```python
from build123d import *

# Parameters (mm, degrees)
SKETCH1_R           = 2.286
BOSS_EXTRUDE1_DEPTH = 12.7
FILLET1_R           = 0.79375


with BuildPart() as part:
    # Sketch1 → Boss-Extrude1 (new body)
    with BuildSketch(Plane(origin=(0, 0, 0), x_dir=(1, 0, 0), z_dir=(0, 1, 0))):
        with BuildLine():
            Line((5.992681083, 6.35), (-5.992681083, 6.35))
            ThreePointArc((-5.992681083, 6.35), (0, -8.73125), (5.992681083, 6.35))
        make_face()
        with Locations(Location((0, 0, 0), (0, 0, 270))):
            Circle(SKETCH1_R, mode=Mode.SUBTRACT)
    extrude(amount=BOSS_EXTRUDE1_DEPTH)

    # Fillet1
    fillet1_edges = [part.edges().sort_by_distance(p)[0] for p in [
        (-5.992681083, 6.35, -6.35),
        (5.992681083, 6.35, -6.35),
        (0, 12.7, 8.73125),
        (0, 12.7, -6.35),
    ]]
    fillet(fillet1_edges, radius=FILLET1_R)


solid = part.part
```
The listing builds one solid part. Answer for the finished solid, in the listing's coordinates (mm). Round coordinates to 2 decimals unless told otherwise and drop trailing zeros. Loops run counter-clockwise (first coordinate to the right, second up) from the corner with the lowest first, then second, coordinate; pieces in that order, holes last. Notation, with made-up numbers: (78, 2.5) - (92, 2.5) arc R17 ccw to (92, 16.5) - close; hole circle Ø11 at (15.5, -15). An arc over 180 degrees is marked (long way). Return JSON: item names as keys, results as strings. Group by question number.
1. Consider probe 1 along X at (y, z) = (4.5, 0); probe 2 along X at (y, z) = (2.5, -0.75); probe 3 along Z at (x, y) = (-1, 2.5). Determine where each line is inside the solid, lowest interval first.
2. Each of these flat-tipped pins is pushed along its axis until it touches: P1, Ø6, axis at y = 4.5, z = -4.5, coming from the -X side; P2, Ø3, axis at x = 0.5, z = -0.5, coming from the -Y side; P3, Ø1, axis at x = -7, y = 9.5, coming from the +Z side; P4, Ø5, axis at y = 9, z = -4, coming from the +X side. Where does it stop, or does it pass through?
3. The part is cut by section B-B on y = 10.25. Determine the outline of the cut face in (x, z).
4. The part is cut by section A-A on x = 0. Determine the outline of the cut face in (y, z).
5. The mould has two halves that part along X. Classify faces 1 (the cylindrical face through (-0.287, 5.87, 8.727)), 2 (the flat face through (0, 6, -6.35)), 3 (the cylindrical face through (-2.03, 6.26, 1.05)): pulls with the +X half, pulls with the -X half, needs draft (parallel to the pull), parting line crosses it, or undercut.
Resolved:
{
 "1": {"probe 1": "x = -8.73 to -2.29, 2.29 to 8.73", "probe 2": "x = -8.7 to -2.16, 2.16 to 8.7", "probe 3": "z = -6.35 to -2.06, 2.06 to 8.67"},
 "2": {"P1": "stops at x = -8.6", "P2": "passes through", "P3": "stops at z = 5.83", "P4": "stops at x = 8.6"},
 "3": {"outline": "(-6.24, -6.11) arc R0.79 ccw to (-5.67, -6.35) - (5.67, -6.35) arc R0.79 ccw to (6.24, -6.11) arc R8.73 ccw (long way) to start; hole circle Ø4.57 at (0, 0)"},
 "4": {"outline": "(0, -6.35) - (11.91, -6.35) arc R0.79 ccw to (12.7, -5.56) - (12.7, -2.29) - (0, -2.29) - close; (0, 2.29) - (12.7, 2.29) - (12.7, 7.94) arc R0.79 ccw to (11.91, 8.73) - (0, 8.73) - close"},
 "5": {"face 1": "parting line crosses it", "face 2": "needs draft", "face 3": "undercut"}
}
